Verification items for the finished model (mm, model axes). A direction names the side the tool comes from. Round coordinates to 2 decimals unless told otherwise and drop trailing zeros. Write each loop counter-clockwise with the first axis right and the second up, starting at its lowest first coordinate (ties: lowest second). Pieces come first, ordered by that corner, then holes. Notation, with made-up numbers: (56.5, 49) - (69.5, 49) arc R24 ccw to (69.5, 65) - close; hole circle Ø10 at (-33, 7). An arc over 180 degrees is marked (long way). Answer as a JSON object with one key per item and string values.
```python
from build123d import *

# Parameters (mm, degrees)
F0_R     = 11
F1_DEPTH = 3.7
F2_R     = 5
F3_DEPTH = 1
F4_R     = 5
F5_DEPTH = 10
F6_R     = 4.5
F7_DEPTH = 14.701
F8_R     = 1.85
F9_DEPTH = 13.701


with BuildPart() as f1:
    # F0 (on Top) → F1 (new body)
    with BuildSketch(Plane.XY):
        Circle(F0_R)
    extrude(amount=F1_DEPTH)

    # F2 (on face) → F3 (join)
    with BuildSketch(Plane.XY.offset(3.7)):
        Circle(F2_R)
    extrude(amount=F3_DEPTH)

    # F4 (on face) → F5 (join)
    with BuildSketch(Plane(origin=(0, 0, 0), x_dir=(1, 0, 0), z_dir=(0, 0, -1))):
        Circle(F4_R)
    extrude(amount=F5_DEPTH)

    # F6 (on face) → F7 (cut, through all)
    with BuildSketch(Plane.XY.offset(4.7)):
        Circle(F6_R)
    extrude(amount=-F7_DEPTH, mode=Mode.SUBTRACT)

    # F8 (on face) → F9 (cut, through all)
    with BuildSketch(Plane.XY.offset(3.7)):
        with Locations((0, 7.75)):
            Circle(F8_R)
        with Locations((-7.75, 0)):
            Circle(F8_R)
        with Locations((0, -7.75)):
            Circle(F8_R)
        with Locations((7.75, 0)):
            Circle(F8_R)
    extrude(amount=-F9_DEPTH, mode=Mode.SUBTRACT)


solid = f1.part
```
Q1. Gauge pin test, flat ends, axial feed: P1, Ø2, axis at x = 7.5, y = 4, coming from the -Z side; P2, Ø4.5, axis at x = 0, y = -7.75, coming from the +Z side; P3, Ø2, axis at x = 7.75, y = 0, coming from the -Z side; P4, Ø3, axis at y = 7.5, z = 0, coming from the +X side. Record the tip position at first contact, or that the pin passes through.
Geometry check:
{"P1": "stops at z = 0", "P2": "stops at z = 3.7", "P3": "passes through", "P4": "stops at x = 9.22"}
Q2. Section check D-D, the plane z = -4.75. Record the cut outline in (x, y).
Geometry check:
{"outline": "circle Ø10 at (0, 0); hole circle Ø9 at (0, 0)"}
Q3. Section check A-A, the plane x = 0. Record the cut outline in (y, z).
Geometry check:
{"outline": "(-11, 0) - (-9.6, 0) - (-9.6, 3.7) - (-11, 3.7) - close; (-5.9, 0) - (-5, 0) - (-5, -10) - (-4.5, -10) - (-4.5, 4.7) - (-5, 4.7) - (-5, 3.7) - (-5.9, 3.7) - close; (4.5, -10) - (5, -10) - (5, 0) - (5.9, 0) - (5.9, 3.7) - (5, 3.7) - (5, 4.7) - (4.5, 4.7) - close; (9.6, 0) - (11, 0) - (11, 3.7) - (9.6, 3.7) - close"}
Q4. Section check C-C, the plane y = -6.5. Record the cut outline in (x, z).
Geometry check:
{"outline": "(-8.87, 0) - (-1.36, 0) - (-1.36, 3.7) - (-8.87, 3.7) - close; (1.36, 0) - (8.87, 0) - (8.87, 3.7) - (1.36, 3.7) - close"}
Q5. Material ranges on line 1 along Y through (x, z) = (0, 2.65); line 2 along Z through (x, y) = (2, 6.5); line 3 along Y through (x, z) = (-1.25, 1.75), recorded low to high. Write a range as [from, to].
Geometry check:
{"line 1": "y = [-11, -9.6], [-5.9, -4.5], [4.5, 5.9], [9.6, 11]", "line 2": "z = [0, 3.7]", "line 3": "y = [-10.93, -9.11], [-6.39, -4.32], [4.32, 6.39], [9.11, 10.93]"}
Q6. Set-up check for faces 1 (the cylindrical face through (-1.08, -4.88, 4.19)), 2 (the flat face through (5, -2, 0)), 3 (the cylindrical face through (-0.59, 4.46, -2.55)): record each of +Z, -Z, +X, -X, +Y, -Y from which the full face is reachable in a straight line by a thin tool's end or side.
Geometry check:
{"face 1": "+Z", "face 2": "-Z", "face 3": "+Z, -Z"}
Q7. Release check for a two-part mould opening along Y. For faces 4 (the flat face through (5, -2, 3.7)), 5 (the cylindrical face through (-2.38, -10.74, 1.82)), 6 (the cylindrical face through (5.9, 0.08, 1.88)), 7 (the cylindrical face through (-0.401, 5.944, 1.876)) record: released by +Y, released by -Y, zero draft, split by the parting line, or undercut.
Geometry check:
{"face 4": "zero draft", "face 5": "split by the parting line", "face 6": "undercut", "face 7": "undercut"}
